from build123d import *

# Parameters (mm, degrees)
F1_DEPTH = 30.48


with BuildPart() as f1:
    # F0 (on Top) → F1 (new body)
    with BuildSketch(Plane.XY):
        with BuildLine():
            ThreePointArc((9.5357191185, 5.50545), (10.6357126807, 2.8498306237), (11.0109, 0))
            ThreePointArc((11.0109, 0), (10.6357126807, -2.8498306237), (9.5357191185, -5.50545))
            Line((9.5357191185, -5.50545), (16.8607351888, -9.73455))
            ThreePointArc((16.8607351888, -9.73455), (23.039686637, -4.7532450387), (30.9627198303, -5.2205619926))
            Line((30.9627198303, -5.2205619926), (41.444029659, 0.8308250585))
            Line((41.444029659, 0.8308250585), (32.4346536017, 6.0323907505))
            ThreePointArc((32.4346536017, 6.0323907505), (23.8499553367, 4.5276117601), (16.8607351888, 9.73455))
            Line((16.8607351888, 9.73455), (9.5357191185, 5.50545))
        make_face()
        with BuildLine():
            ThreePointArc((0, 11.0109), (5.50545, 9.5357191185), (9.5357191185, 5.50545))
            Line((9.5357191185, 5.50545), (16.8607351888, 9.73455))
            ThreePointArc((16.8607351888, 9.73455), (15.6362742725, 17.5763314035), (20.0024992228, 24.204220947))
            Line((20.0024992228, 24.204220947), (20.0024992228, 36.3069950492))
            Line((20.0024992228, 36.3069950492), (10.9931231654, 31.1054293572))
            ThreePointArc((10.9931231654, 31.1054293572), (11.0064548941, 30.7928409727), (11.0109, 30.48))
            ThreePointArc((11.0109, 30.48), (7.785882057, 22.694117943), (0, 19.4691))
            Line((0, 19.4691), (0, 11.0109))
        make_face()
        with BuildLine():
            Line((16.8607351888, -9.73455), (9.5357191185, -5.50545))
            ThreePointArc((9.5357191185, -5.50545), (5.50545, -9.5357191185), (0, -11.0109))
            Line((0, -11.0109), (0, -19.4691))
            ThreePointArc((0, -19.4691), (7.4034123646, -22.3295764423), (10.9602206075, -29.4247829396))
            Line((10.9602206075, -29.4247829396), (21.4415304363, -35.4761699907))
            Line((21.4415304363, -35.4761699907), (21.4415304363, -25.0730386068))
            ThreePointArc((21.4415304363, -25.0730386068), (15.8460044711, -18.3908613207), (16.8607351888, -9.73455))
        make_face()
        with BuildLine():
            ThreePointArc((-9.5357191185, 5.50545), (-5.50545, 9.5357191185), (0, 11.0109))
            Line((0, 11.0109), (0, 19.4691))
            ThreePointArc((0, 19.4691), (-7.4034123646, 22.3295764423), (-10.9602206075, 29.4247829396))
            Line((-10.9602206075, 29.4247829396), (-21.4415304363, 35.4761699907))
            Line((-21.4415304363, 35.4761699907), (-21.4415304363, 25.0730386068))
            ThreePointArc((-21.4415304363, 25.0730386068), (-17.0210052498, 21.0141556767), (-15.3855543073, 15.24))
            ThreePointArc((-15.3855543073, 15.24), (-15.7607416267, 12.3901693763), (-16.8607351888, 9.73455))
            Line((-16.8607351888, 9.73455), (-9.5357191185, 5.50545))
        make_face()
        with BuildLine():
            Line((0, -19.4691), (0, -11.0109))
            ThreePointArc((0, -11.0109), (-5.50545, -9.5357191185), (-9.5357191185, -5.50545))
            Line((-9.5357191185, -5.50545), (-16.8607351888, -9.73455))
            ThreePointArc((-16.8607351888, -9.73455), (-15.7607416267, -12.3901693763), (-15.3855543073, -15.24))
            ThreePointArc((-15.3855543073, -15.24), (-16.6076055791, -20.2816623632), (-20.0024992228, -24.204220947))
            Line((-20.0024992228, -24.204220947), (-20.0024992228, -36.3069950492))
            Line((-20.0024992228, -36.3069950492), (-10.9931231654, -31.1054293572))
            ThreePointArc((-10.9931231654, -31.1054293572), (-8.0039508656, -22.9184730808), (0, -19.4691))
        make_face()
        with BuildLine():
            ThreePointArc((-9.5357191185, -5.50545), (-11.0109, 0), (-9.5357191185, 5.50545))
            Line((-9.5357191185, 5.50545), (-16.8607351888, 9.73455))
            ThreePointArc((-16.8607351888, 9.73455), (-23.039686637, 4.7532450387), (-30.9627198303, 5.2205619926))
            Line((-30.9627198303, 5.2205619926), (-41.444029659, -0.8308250585))
            Line((-41.444029659, -0.8308250585), (-32.4346536017, -6.0323907505))
            ThreePointArc((-32.4346536017, -6.0323907505), (-23.8499553367, -4.5276117601), (-16.8607351888, -9.73455))
            Line((-16.8607351888, -9.73455), (-9.5357191185, -5.50545))
        make_face()
        with BuildLine():
            Line((20.0024992228, 36.3069950492), (20.0024992228, 24.204220947))
            ThreePointArc((20.0024992228, 24.204220947), (31.4381166706, 25.0288487283), (37.4073543073, 15.24))
            ThreePointArc((37.4073543073, 15.24), (36.0847443376, 10.0077007826), (32.4346536017, 6.0323907505))
            Line((32.4346536017, 6.0323907505), (41.444029659, 0.8308250585))
            Line((41.444029659, 0.8308250585), (48.509925581, 4.9103219711))
            Line((48.509925581, 4.9103219711), (27.7879107515, 40.8019044911))
            Line((27.7879107515, 40.8019044911), (20.0024992228, 36.3069950492))
        make_face()
        with BuildLine():
            Line((41.444029659, 0.8308250585), (30.9627198303, -5.2205619926))
            ThreePointArc((30.9627198303, -5.2205619926), (35.6570863553, -9.2834395091), (37.4073543073, -15.24))
            ThreePointArc((37.4073543073, -15.24), (32.1706099841, -24.6154490576), (21.4415304363, -25.0730386068))
            Line((21.4415304363, -25.0730386068), (21.4415304363, -35.4761699907))
            Line((21.4415304363, -35.4761699907), (28.5074263583, -39.5556669033))
            Line((28.5074263583, -39.5556669033), (49.2294411878, -3.6640843834))
            Line((49.2294411878, -3.6640843834), (41.444029659, 0.8308250585))
        make_face()
        with BuildLine():
            Line((-21.4415304363, 35.4761699907), (-10.9602206075, 29.4247829396))
            ThreePointArc((-10.9602206075, 29.4247829396), (-0.8404842294, 41.4587752081), (10.9931231654, 31.1054293572))
            Line((10.9931231654, 31.1054293572), (20.0024992228, 36.3069950492))
            Line((20.0024992228, 36.3069950492), (20.0024992228, 44.4659888744))
            Line((20.0024992228, 44.4659888744), (-21.4415304363, 44.4659888744))
            Line((-21.4415304363, 44.4659888744), (-21.4415304363, 35.4761699907))
        make_face()
        with BuildLine():
            Line((21.4415304363, -35.4761699907), (10.9602206075, -29.4247829396))
            ThreePointArc((10.9602206075, -29.4247829396), (10.9982228541, -29.9517833197), (11.0109, -30.48))
            ThreePointArc((11.0109, -30.48), (0.3128409727, -41.4864548941), (-10.9931231654, -31.1054293572))
            Line((-10.9931231654, -31.1054293572), (-20.0024992228, -36.3069950492))
            Line((-20.0024992228, -36.3069950492), (-20.0024992228, -44.4659888744))
            Line((-20.0024992228, -44.4659888744), (21.4415304363, -44.4659888744))
            Line((21.4415304363, -44.4659888744), (21.4415304363, -35.4761699907))
        make_face()
        with BuildLine():
            Line((-41.444029659, -0.8308250585), (-30.9627198303, 5.2205619926))
            ThreePointArc((-30.9627198303, 5.2205619926), (-36.3245946547, 20.0015069099), (-21.4415304363, 25.0730386068))
            Line((-21.4415304363, 25.0730386068), (-21.4415304363, 35.4761699907))
            Line((-21.4415304363, 35.4761699907), (-28.5074263583, 39.5556669033))
            Line((-28.5074263583, 39.5556669033), (-49.2294411878, 3.6640843834))
            Line((-49.2294411878, 3.6640843834), (-41.444029659, -0.8308250585))
        make_face()
        with BuildLine():
            ThreePointArc((-20.0024992228, -24.204220947), (-35.4841104253, -21.4572682982), (-32.4346536017, -6.0323907505))
            Line((-32.4346536017, -6.0323907505), (-41.444029659, -0.8308250585))
            Line((-41.444029659, -0.8308250585), (-48.509925581, -4.9103219711))
            Line((-48.509925581, -4.9103219711), (-27.7879107515, -40.8019044911))
            Line((-27.7879107515, -40.8019044911), (-20.0024992228, -36.3069950492))
            Line((-20.0024992228, -36.3069950492), (-20.0024992228, -24.204220947))
        make_face()
    extrude(amount=F1_DEPTH)


solid = f1.part
Geometry check sheet. Reference: the model listing, model coordinates, mm. A direction names the side the tool comes from. Give positions to 0.01 mm unless a question says otherwise; leave off trailing zeros. Loops run counter-clockwise (first coordinate to the right, second up) from the corner with the lowest first, then second, coordinate; pieces in that order, holes last. Notation, with made-up numbers: M 88,-23.5 L 142,-23.5 A24 ccw 142,-3.5 Z; hole C 79,-39.75 d1. An arc over 180 degrees is marked long. Answer as a JSON object with one key per item and string values. Group by question number.
Item 1: Access from +Z, -Z, +X, -X, +Y, -Y to the whole of each face (thin tool, end or side, straight path). Record for faces 1 (the flat face through (44.928, 2.842, 15.027)), 2 (the flat face through (-20.002, -40, 15)), 3 (the flat face through (23.95, 38.586, 15.027)), 4 (the flat face through (-12, 1, 30.48)).
Item 2: Gauge pin test, flat ends, axial feed: pin 1 (8 mm diameter, centred on y = 28, z = 27, fed in from +X); pin 2 (7 mm diameter, centred on y = -38, z = 13, fed in from +X); pin 3 (12 mm diameter, centred on x = -28.5, z = 25, fed in from +Y). Record the tip position at first contact, or that the pin passes through.
Item 3: Mould release check, pull along X, two halves, no side actions. Record for faces 5 (the flat face through (0, 44.466, 15)), 6 (the flat face through (-24.93, 37.49, 15.03)), 7 (the flat face through (-45.391, 1.448, 15.027)): pulls with the +X half, pulls with the -X half, needs draft (parallel to the pull), parting line crosses it, or undercut.
Item 4: Sectioned sample at A-A on x = -5. Record the boundary of the cut face in (y, z).
Item 5: Sectioned sample at B-B on z = 24. Record the boundary of the cut face in (x, y), plus the area to 3 significant figures.
Item 6: Material ranges on L1, parallel to X at y = -37, z = 26; L2, parallel to X at y = 21, z = 4; L3, parallel to X at y = 17, z = 21.5, recorded low to high.
Findings below:
{
 "1": {"face 1": "+Z, -Z, +X", "face 2": "+Z, -Z, -Y", "face 3": "+Z, -Z, +Y", "face 4": "+Z, +X, -X, +Y, -Y"},
 "2": {"pin 1": "x = 37.49", "pin 2": "x = 31.43", "pin 3": "y = 39.56"},
 "3": {"face 5": "needs draft", "face 6": "undercut", "face 7": "pulls with the -X half"},
 "4": {"outline": "M -44.47,0 L -40.29,0 L -40.29,30.48 L -44.47,30.48 Z; M -20.67,0 L -9.81,0 L -9.81,30.48 L -20.67,30.48 Z; M 9.81,0 L 20.67,0 L 20.67,30.48 L 9.81,30.48 Z; M 40.29,0 L 44.47,0 L 44.47,30.48 L 40.29,30.48 Z"},
 "5": {"outline": "M -49.23,3.66 L -41.44,-0.83 L -48.51,-4.91 L -27.79,-40.8 L -20,-36.31 L -20,-44.47 L 21.44,-44.47 L 21.44,-35.48 L 28.51,-39.56 L 49.23,-3.66 L 41.44,0.83 L 48.51,4.91 L 27.79,40.8 L 20,36.31 L 20,44.47 L -21.44,44.47 L -21.44,35.48 L -28.51,39.56 Z; hole C -26.4,-15.24 d22.02; hole C -26.4,15.24 d22.02; hole C 0,-30.48 d22.02; hole C 0,0 d22.02; hole C 0,30.48 d22.02; hole C 26.4,-15.24 d22.02; hole C 26.4,15.24 d22.02", "area": "3,930 mm2"},
 "6": {"L1": "-29.98 to -21.2, -20 to -8.87, 8.87 to 21.44, 24.08 to 29.98", "L2": "-39.22 to -35.78, -17.01 to -5.6, 5.6 to 17.01, 35.78 to 39.22", "L3": "-41.53 to -37.27, -15.53 to 15.53, 37.27 to 41.53"}
}
